Check sheet for the modelled part. Datum: model origin and axes. Units: mm. Face numbers are marked on the shaded views. Round coordinates to 2 decimals unless told otherwise and drop trailing zeros. Order: outer loops, then holes, each group sorted by start corner. A loop starts at its lowest first (then second) coordinate and runs counter-clockwise, first axis right, second up.
Q1. Depth check by flat-ended pin: P1, Ø4, axis at x = 22, y = -15.5, coming from the +Z side; P2, Ø1, axis at y = -8, z = 18.5, coming from the -X side; P3, Ø10, axis at x = 0, z = 63.5, coming from the +Y side; P4, Ø5, axis at y = -15, z = 77.5, coming from the -X side. Enter the tip coordinate at first touch or a pass-through.
Q2. Cross-section at A-A on y = -16. Give the number of separate pieces and of enclosed holes in the cut face, then the cut area to 3 significant figures.
Q3. Cross-section at C-C on z = 54. Record the cut outline in (x, y).
Q4. Cross-section at B-B on z = 21.5. Record the cut outline in (x, y).
Q5. Mould release check, pull along Z, two halves, no side actions. Record for the marked faces 1, 2 and 3: +Z half, -Z half, draft (parallel to the pull), parting line (faces both ways), or undercut.
Q6. Scan lines: probe 1 along Z at (x, y) = (1, -11.75); probe 2 along Z at (x, y) = (45.5, -5); probe 3 along Z at (x, y) = (-8.5, -23.25). Record each from-to range of solid material in increasing order.
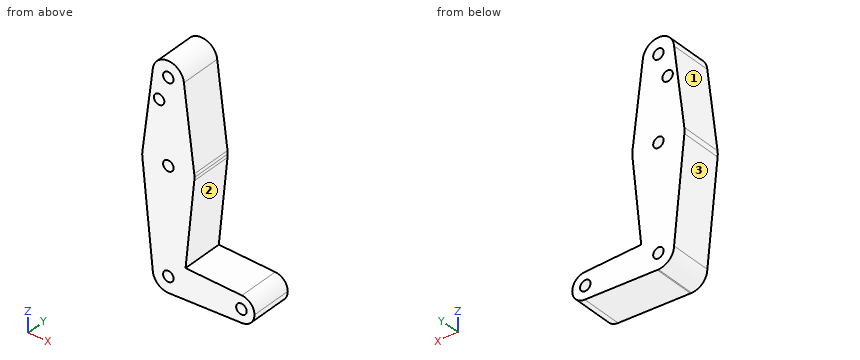
from build123d import *

# Parameters (mm, degrees)
F0_R     = 3.175
F1_DEPTH = 25.4


with BuildPart() as f1:
    # F0 (on Front) → F1 (new body)
    with BuildSketch(Plane.XZ):
        with BuildLine():
            Line((0.6773435479, 9.500885786), (0, 9.525))
            ThreePointArc((0, 9.525), (-6.7351920908, 6.7351920908), (-9.525, 0))
            ThreePointArc((-9.525, 0), (-6.7351920908, -6.7351920908), (0, -9.525))
            Line((0, -9.525), (0.6773435479, -9.500885786))
            ThreePointArc((0.6773435479, -9.500885786), (6.9705567315, -6.4912990883), (9.525, 0))
            ThreePointArc((9.525, 0), (6.9705567315, 6.4912990883), (0.6773435479, 9.500885786))
        make_face()
        Circle(F0_R, mode=Mode.SUBTRACT)
        with BuildLine():
            ThreePointArc((-9.525, 0), (-6.7351920908, 6.7351920908), (0, 9.525))
            ThreePointArc((0, 9.525), (0.3388863295, 9.5189695375), (0.6773435479, 9.500885786))
            Line((0.6773435479, 9.500885786), (10.4513434813, 9.1529200793))
            Line((10.4513434813, 9.1529200793), (15.7522627132, 61.5297015358))
            ThreePointArc((15.7522627132, 61.5297015358), (-0.1865159815, 47.6260958159), (-15.7941956396, 61.9003822774))
            Line((-15.7941956396, 61.9003822774), (-9.525, 0))
        make_face()
        with BuildLine():
            Line((10.4513434813, 9.1529200793), (0.6773435479, 9.500885786))
            ThreePointArc((0.6773435479, 9.500885786), (6.9705567315, 6.4912990883), (9.525, 0))
            Line((9.525, 0), (10.4513434813, 9.1529200793))
        make_face()
        with BuildLine():
            Line((0.6773435479, -9.500885786), (0, -9.525))
            ThreePointArc((0, -9.525), (0.3388863295, -9.5189695375), (0.6773435479, -9.500885786))
        make_face()
        with BuildLine():
            ThreePointArc((-15.7498007105, 65.4897665669), (-15.8737785304, 63.696333282), (-15.7941956396, 61.9003822774))
            ThreePointArc((-15.7941956396, 61.9003822774), (-0.1865159815, 47.6260958159), (15.7522627132, 61.5297015358))
            ThreePointArc((15.7522627132, 61.5297015358), (15.8442914769, 62.5129409485), (15.8750073521, 63.5))
            ThreePointArc((15.8750073521, 63.5), (15.8438216155, 64.494572565), (15.7503869317, 65.4852375421))
            ThreePointArc((15.7503869317, 65.4852375421), (0.0022898231, 79.3749998359), (-15.7498007105, 65.4897665669))
        make_face()
        with Locations((7.3521e-06, 63.5)):
            Circle(F0_R, mode=Mode.SUBTRACT)
        with BuildLine():
            Line((10.4513434813, 9.1529200793), (9.525, 0))
            ThreePointArc((9.525, 0), (6.9705567315, -6.4912990883), (0.6773435479, -9.500885786))
            Line((0.6773435479, -9.500885786), (44.7324052746, -7.9324746146))
            ThreePointArc((44.7324052746, -7.9324746146), (36.5125, 0), (44.7324052746, 7.9324746146))
            Line((44.7324052746, 7.9324746146), (10.4513434813, 9.1529200793))
        make_face()
        with BuildLine():
            Line((-9.5046001494, 114.9230577828), (-15.7498007105, 65.4897665669))
            ThreePointArc((-15.7498007105, 65.4897665669), (0.0022898231, 79.3749998359), (15.7503869317, 65.4852375421))
            Line((15.7503869317, 65.4852375421), (9.4761320574, 115.2636110372))
            ThreePointArc((9.4761320574, 115.2636110372), (9.5127751694, 114.782424685), (9.525, 114.3))
            ThreePointArc((9.525, 114.3), (-0.3116958272, 104.7801013287), (-9.5046001494, 114.9230577828))
        make_face()
        with Locations((-5.6031434797, 99.3416681886)):
            Circle(F0_R, mode=Mode.SUBTRACT)
        with BuildLine():
            ThreePointArc((52.3875, 0), (50.1616327839, 5.5119104847), (44.7324052746, 7.9324746146))
            ThreePointArc((44.7324052746, 7.9324746146), (36.5125, 0), (44.7324052746, -7.9324746146))
            ThreePointArc((44.7324052746, -7.9324746146), (50.1616327839, -5.5119104847), (52.3875, 0))
        make_face()
        with Locations((44.45, 0)):
            Circle(F0_R, mode=Mode.SUBTRACT)
        with BuildLine():
            ThreePointArc((9.4761320574, 115.2636110372), (-0.1708705294, 123.8234672395), (-9.5046001494, 114.9230577828))
            ThreePointArc((-9.5046001494, 114.9230577828), (-0.3116958272, 104.7801013287), (9.525, 114.3))
            ThreePointArc((9.525, 114.3), (9.5127751694, 114.782424685), (9.4761320574, 115.2636110372))
        make_face()
        with Locations((0, 114.3)):
            Circle(F0_R, mode=Mode.SUBTRACT)
    extrude(amount=F1_DEPTH)


solid = f1.part
Results found:
1. P1: stops at z = 8.81
1. P2: stops at x = -11.45
1. P3: stops at y = 0
1. P4: stops at x = -14.55
2. separate pieces: 1
2. enclosed holes: 6
2. area: 3,760 mm2
3. outline: (-14.99, -25.4) - (14.99, -25.4) - (14.99, 0) - (-14.99, 0) - close
4. outline: (-11.7, -25.4) - (11.7, -25.4) - (11.7, 0) - (-11.7, 0) - close
5. face 1: +Z half
5. face 2: undercut
5. face 3: -Z half
6. probe 1: z = -9.49 to -3.01, 3.01 to 60.49, 66.51 to 111.29, 117.31 to 123.77
6. probe 2: z = -7.87 to -3, 3 to 7.87
6. probe 3: z = -4.3 to 98.04, 100.64 to 118.6
